Verification items for the finished model (mm, model axes). A direction names the side the tool comes from. Coordinates: 2 decimals unless noted, no trailing zeros. Loops run counter-clockwise (first coordinate to the right, second up) from the corner with the lowest first, then second, coordinate; pieces in that order, holes last. Notation, with made-up numbers: (-32, 30.25) - (10, 30.25) arc R28 cw to (10, 52.25) - close; hole circle Ø10 at (40, 59.5). An arc over 180 degrees is marked (long way). Answer as CSV lines item,"result". Start each with the question number.
1. Gauge pin test, flat ends, axial feed: P1, Ø0.5, axis at y = 13, z = -53, coming from the +X side; P2, Ø1.8, axis at x = -101.5, y = 12, coming from the -Z side. Record the tip position at first contact, or that the pin passes through.
2. Set-up check for faces 1 (the flat face through (-100, 17.475, -55)), 2 (the flat face through (-98, 10, -53.863)), 3 (the flat face through (-102.413, 10, -56)): record each of +Z, -Z, +X, -X, +Y, -Y from which the full face is reachable in a straight line by a thin tool's end or side.
3. Release check for a two-part mould opening along X. For faces 4 (the cylindrical face through (-100.47, 9.99, -57.89)), 5 (the flat face through (-102, 10, -52.857)), 6 (the cylindrical face through (-102.7, 9.987, -57.883)), 7 (the cylindrical face through (-104.06, 10.19, -57.88)) record: pulls with the +X half, pulls with the -X half, needs draft (parallel to the pull), parting line crosses it, or undercut.
4. Material ranges on line 1 (X direction, y = 15.5, z = -53.55); line 2 (Z direction, x = -99, y = 4); line 3 (X direction, y = 16.75, z = -56.9), recorded low to high. Write a range as [from, to].
5. Cross-section at A-A (z = -57.7). Enter the section's corners in (x, y).
6. Cross-section at B-B (y = 7.75). Enter the section's corners in (x, z).
7. Cross-section at C-C (x = -102.25). Enter the section's corners in (y, z), plus the area to 3 significant figures.
8. Cross-section at D-D (z = -55). Enter the section's corners in (x, y).
Solid Edge part; units mm, degrees
sketch "Sketch1" plane through (-38.046, 17.4752, -58.1274) normal (0, -1, 0) x (1, 0, 0)
  line L0 (-62.7158, 3.9492) -> (-62.7158, -0.064)
  line L1 (-62.7158, -0.064) -> (-56.1372, -0.064)
  line L2 (-56.1372, 5.27) -> (-56.1372, -0.064)
  line L3 (-66.2972, 5.27) -> (-56.1372, 5.27)
  line L4 (-66.2972, -0.064) -> (-66.2972, 5.27)
  line L5 (-66.2972, -0.064) -> (-64.3668, -0.064)
  line L6 (-64.3668, -0.064) -> (-64.3668, 3.9492)
  line L7 (-64.3668, 3.9492) -> (-62.7158, 3.9492)
extrude "Protrusion1" add sketch "Sketch1" along normal up to surface (14.7701 mm away)
sketch "Sketch2" plane through (-38.046, 17.4752, -58.1274) normal (0, -1, 0) x (1, 0, 0)
  circle A0 centre (-54.664, 0.1392) radius 5.0038
extrude "Cutout1" cut sketch "Sketch2" along normal through all
sketch "Sketch3" plane through (-38.046, 17.4752, -58.1274) normal (0, -1, 0) x (1, 0, 0)
  line L0 (-61.5982, 5.27) -> (-61.5982, 4.2646)
  line L1 (-61.5982, 4.2646) -> (-56.1372, 4.2646)
  line L2 (-56.1372, 4.2646) -> (-56.1372, 5.27)
  line L3 (-56.1372, 5.27) -> (-61.5982, 5.27)
extrude "Cutout2" cut sketch "Sketch3" along normal through all
fillet "Round_1" radius 1.016 3 edges at (-100.7618, 10.0901, -58.1914) (-102.4128, 10.0901, -58.1914) (-104.3432, 10.0901, -58.1914)
properties material "Gold"
Values follow:
1,P1,"stops at x = -99.64"
1,P2,"stops at z = -57.73"
2,face 1,"+Z, -Z, +X, -X, +Y"
2,face 2,"+Z, +X, +Y, -Y"
2,face 3,"-Z, +Y, -Y"
3,face 4,"undercut"
3,face 5,"needs draft"
3,face 6,"undercut"
3,face 7,"pulls with the -X half"
4,line 1,"x = [-104.34, -99.64]"
4,line 2,"z = [-58.19, -53.86]"
4,line 3,"x = [-104.34, -102.41], [-100.76, -97.59]"
5,outline,"(-104.2, 2.71) - (-102.56, 2.71) - (-102.56, 17.48) - (-104.2, 17.48) - close; (-100.62, 2.71) - (-97.71, 2.71) - (-97.71, 17.48) - (-100.62, 17.48) - close"
6,outline,"(-104.34, -57.18) arc R1.02 ccw to (-103.38, -58.19) arc R1.02 ccw to (-102.41, -57.18) - (-102.41, -54.18) - (-100.76, -54.18) - (-100.76, -57.18) arc R1.02 ccw to (-99.75, -58.19) - (-97.71, -58.19) arc R5 cw to (-95.54, -53.86) - (-99.64, -53.86) - (-99.64, -52.86) - (-104.34, -52.86) - close"
7,outline,"(2.71, -54.18) - (17.48, -54.18) - (17.48, -52.86) - (2.71, -52.86) - close"
7,area,"19.5 mm²"
8,outline,"(-104.34, 2.71) - (-102.41, 2.71) - (-102.41, 17.48) - (-104.34, 17.48) - close; (-100.76, 2.71) - (-96.72, 2.71) - (-96.72, 17.48) - (-100.76, 17.48) - close"
